Part model, mm, in its own coordinate system. A direction names the side the tool comes from. Coordinates: 2 decimals unless noted, no trailing zeros. Order: outer loops, then holes, each group sorted by start corner. A loop starts at its lowest first (then second) coordinate and runs counter-clockwise, first axis right, second up.
1) Wall check: L1, parallel to X at y = 34.5, z = 95; L2, parallel to Y at x = -3.5, z = 194.5; L3, parallel to X at y = -35.5, z = 119. Give the ranges that are in metal, low to high.
2) Cut at C-C (z = 107.5). List the corners of the cut face in (x, y), and give its area (3 significant figures).
3) Tool access for faces 1 (the flat face through (0, -37, 156)), 2 (the cylindrical face through (38.196, 38.289, 157.325)): list every direction of +Z, -Z, +X, -X, +Y, -Y with a clear straight run to the whole face (end or side of a thin tool).
4) Cut at A-A (y = 20). List the corners of the cut face in (x, z), and give its area (3 significant figures).
5) Cut at B-B (x = -14). List the corners of the cut face in (y, z).
Autodesk Inventor part; units mm, degrees
ref_plane "Start plane" through (0, 0, 0) normal (0, 0, 1) x (1, 0, 0)
ref_plane "End plane" through (0, 0, 1000) normal (0, 0, 1) x (1, 0, 0)
ref_plane "YZ Plane" through (0, 0, 0) normal (1, 0, 0) x (0, 1, 0)
ref_plane "Start plane" through (0, 0, 0) normal (0, 0, 1) x (1, 0, 0)
ref_plane "End plane" through (0, 0, 1000) normal (0, 0, 1) x (1, 0, 0)
sketch "Sketch" plane through (0, 0, 0) normal (0, 0, 1) x (1, 0, 0)
  line L0 (-40, -34) -> (-40, 34)
  line L1 (-34, 40) -> (34, 40)
  line L2 (40, 34) -> (40, -34)
  line L3 (34, -40) -> (-34, -40)
  arc A0 (-40, -34) -> (-34, -40) centre (-34, -34) ccw
  arc A1 (40, 34) -> (34, 40) centre (34, 34) ccw
  arc A2 (-34, 40) -> (-40, 34) centre (-34, 34) ccw
  arc A3 (34, -40) -> (40, -34) centre (34, -34) ccw
  arc A4 (-34, 37) -> (-37, 34) centre (-34, 34) ccw
  line L4 (-34, 37) -> (34, 37)
  arc A5 (37, 34) -> (34, 37) centre (34, 34) ccw
  line L5 (37, 34) -> (37, -34)
  arc A6 (34, -37) -> (37, -34) centre (34, -34) ccw
  line L6 (34, -37) -> (-34, -37)
  arc A7 (-37, -34) -> (-34, -37) centre (-34, -34) ccw
  line L7 (-37, -34) -> (-37, 34)
  line L8 (0, 57.7397) -> (0, -57.7397) construction
  line L9 (-57.7397, 0) -> (57.7397, 0) construction
  dimension "d7" = 6
  dimension "d9" = 80
  dimension "d11" = 80
  dimension "d12" = 3
  dimension "d15" = 40
  dimension "d16" = 40
extrude "Body" add sketch "Sketch" along normal up to surface (1000 mm away) from surface at 0
sketch "Sketch3" plane through (0, 0, 0) normal (0, 0, 1) x (1, 0, 0)
  line L0 (0, 0) -> (10, 0)
ref_plane "Work Plane3" through (0, 0, 0) normal (0, -1, 0) x (1, 0, 0)
sketch "Sketch7" plane through (0, 0, 0) normal (0, 1, 0) x (-1, 0, 0)
  line L0 (40, 0) -> (40, 1000)
  line L1 (-40, 0) -> (-40, 1000)
  line L2 (40, 290) -> (-40, 319.1176)
  line L3 (-40, 1000) -> (-34, 1000)
  line L4 (40, 1000) -> (-40, 1000)
  point P0 (0, 0)
  dimension "d37" = 290
  dimension "d38" = 70
extrude "Extrusion3" cut sketch "Sketch7" along normal through all both and the other way through all
sketch "Sketch4" plane through (0, 0, 0) normal (0, -1, 0) x (1, 0, 0)
  line L0 (-2, 0) -> (12, 0)
  line L1 (-2, 1000) -> (12, 1000)
  dimension "d18" = 1000
equation "\"d7\" = G_IR"
equation "\"d9\" = G_W"
equation "\"d11\" = G_H"
equation "\"d12\" = G_T"
equation "\"d15\" = 0.5 * d9"
equation "\"d16\" = 0.5 * d11"
equation "\"d3\" = G_L"
equation "\"G_W\" = 80"
equation "\"G_H\" = 80"
equation "\"G_T\" = 3"
equation "\"G_IR\" = 6"
equation "\"G_L\" = d18"
equation "\"G_OFFSET_START\" = 0"
equation "\"G_OFFSET_END\" = 0"
properties part number "PRS 940-91 Leg tube" material "Steel, Mild"
Geometry check:
1. L1: x = -39.98 to -36.96, 36.96 to 39.98
1. L2: y = -40 to -37, 37 to 40
1. L3: x = -39.81 to -36.6, 36.6 to 39.81
2. outline: (-40, -34) arc R6 ccw to (-34, -40) - (34, -40) arc R6 ccw to (40, -34) - (40, 34) arc R6 ccw to (34, 40) - (-34, 40) arc R6 ccw to (-40, 34) - close; hole (-37, -34) arc R3 ccw to (-34, -37) - (34, -37) arc R3 ccw to (37, -34) - (37, 34) arc R3 ccw to (34, 37) - (-34, 37) arc R3 ccw to (-37, 34) - close
2. area: 901 mm2
3. face 1: +Z, -Z
3. face 2: +Z, -Z, +X, +Y
4. outline: (-40, 0) - (-37, 0) - (-37, 291.09) - (-40, 290) - close; (37, 0) - (40, 0) - (40, 319.12) - (37, 318.03) - close
4. area: 1,830 mm2
5. outline: (-40, 0) - (-37, 0) - (-37, 299.46) - (-40, 299.46) - close; (37, 0) - (40, 0) - (40, 299.46) - (37, 299.46) - close
